Job drawing, mm, ordinate dimensions from the low corner. One solid piece. A direction names the side the tool comes from. Give positions to 0.01 mm unless a question says otherwise; leave off trailing zeros. Write each loop counter-clockwise with the first axis right and the second up, starting at its lowest first coordinate (ties: lowest second). Pieces come first, ordered by that corner, then holes. Notation, with made-up numbers: M 62.25,51 L 115.25,51 A14 cw 115.25,73 Z; hole C 88.25,88.25 d10. An arc over 180 degrees is marked long. Answer as CSV lines item,"result". Start each with the question number.
1) Slice it at C-C, the plane y = 391. Give the cut face in (x, z), plus the area to 3 significant figures.
2) Slice it at A-A, the plane z = 235.5. Give the cut face in (x, y).
3) Tool access for the marked faces 1 and 2: list every direction of +Z, -Z, +X, -X, +Y, -Y with a clear straight run to the whole face (end or side of a thin tool).
4) Pin check, flat tips, straight feed: pin 1 Ø12.5 at (x, z) = (159, 16) entering from -Y; pin 2 Ø5 at (x, y) = (218.5, 188) entering from +Z; pin 3 Ø8 at (y, z) = (689, 53.5) entering from -X; pin 4 Ø15 at (x, z) = (21.5, 330) entering from +Y. Stop position of each tip, or through.
5) Mould opens along X. For the marked faces 3, 4, 5 and 6 say: pulls with the +X half, pulls with the -X half, needs draft (parallel to the pull), parting line crosses it, or undercut.
6) Slice it at B-B, the plane x = 28.5. Give the cut face in (y, z), plus the area to 3 significant figures.
7) Slice it at D-D, the plane x = 106. Give the cut face in (y, z).
8) Wall check: line 1 along Y through (x, z) = (378.5, 141); line 2 along Z through (x, y) = (55.5, 540). Give the ranges that are in metal, low to high. Write a range as from..to.
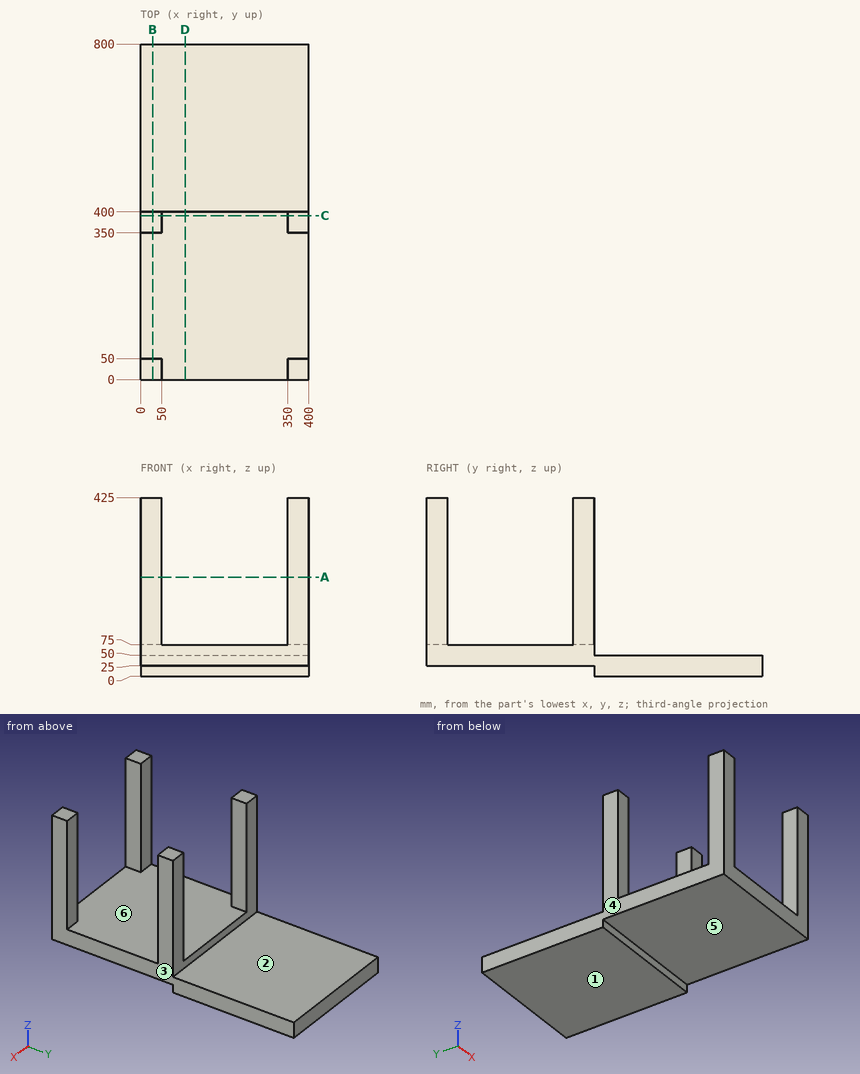
Found:
1,outline,"M 0,25 L 400,25 L 400,425 L 350,425 L 350,75 L 50,75 L 50,425 L 0,425 Z"
1,area,"55,000 mm²"
2,outline,"M 0,0 L 50,0 L 50,50 L 0,50 Z; M 0,350 L 50,350 L 50,400 L 0,400 Z; M 350,0 L 400,0 L 400,50 L 350,50 Z; M 350,350 L 400,350 L 400,400 L 350,400 Z"
3,face 1,"-Z, +X, -X, +Y, -Y"
3,face 2,"+Z, +X, -X, +Y"
4,pin 1,"y = 400"
4,pin 2,"z = 75"
4,pin 3,"x = 0"
4,pin 4,"y = 400"
5,face 3,"pulls with the +X half"
5,face 4,"pulls with the -X half"
5,face 5,"needs draft"
5,face 6,"undercut"
6,outline,"M 0,25 L 400,25 L 400,0 L 800,0 L 800,50 L 400,50 L 400,425 L 350,425 L 350,75 L 50,75 L 50,425 L 0,425 Z"
6,area,"75,000 mm²"
7,outline,"M 0,25 L 400,25 L 400,0 L 800,0 L 800,50 L 400,50 L 400,75 L 0,75 Z"
8,line 1,"0..50, 350..400"
8,line 2,"0..50"
